Verification items for the finished model (mm, model axes). A direction names the side the tool comes from. Give positions to 0.01 mm unless a question says otherwise; leave off trailing zeros. Write each loop counter-clockwise with the first axis right and the second up, starting at its lowest first coordinate (ties: lowest second). Pieces come first, ordered by that corner, then holes. Notation, with made-up numbers: (33, 84.5) -> (42, 84.5) arc R8 ccw to (42, 93.5) -> close; hole circle Ø7 at (-20, 58). An arc over 180 degrees is marked (long way). Use one line per item in the form item = value. Start each with the question number.
(1) Scan lines: L1, parallel to Y at x = -99.5, z = 10; L2, parallel to X at y = 42.5, z = -20; L3, parallel to Y at x = -99.5, z = 5. Record each from-to range of solid material in increasing order.
(2) Section check B-B, the plane z = -13. State how many separate pieces and enclosed holes the cut face has, plus the area to 3 significant figures.
(3) Depth check by flat-ended pin: pin 1 Ø6 at (y, z) = (33, 0.5) entering from +X; pin 2 Ø2.5 at (x, y) = (-83, 42) entering from -Z; pin 3 Ø5 at (x, z) = (-104.5, 2) entering from +Y; pin 4 Ø2.5 at (y, z) = (43.5, -14) entering from +X. Enter the tip coordinate at first touch or a pass-through.
(4) Set-up check for faces 4 (the face through (-76.171, 42, -17)), 5 (the face through (-88.35, 42.46, 9.86)), 6 (the face through (-64.993, 4.014, -11.003)), 7 (the face through (-104, 2, 8.376)), 8 (the face through (-83, 43, -23.267)): record each of +Z, -Z, +X, -X, +Y, -Y from which the full face is reachable in a straight line by a thin tool's end or side.
(5) Section check D-D, the plane y = 42. Record the cut outline in (x, z).
(6) Release check for a two-part mould opening along Y. For faces 1 (the face through (-66, 3, -14)), 2 (the face through (-103, 2, 13.376)), 3 (the face through (-82, 0, -3)) record: pulls with the +Y half, pulls with the -Y half, needs draft (parallel to the pull), parting line crosses it, or undercut.
from build123d import *

# Parameters (mm, degrees)
AUFSATZ_LINEAR_AUSTRAGEN1_DEPTH  = 5
VERRUNDUNG1_RADIUS               = 2.5
VERRUNDUNG1_LENGTH               = 5
SKIZZE6_W                        = 37
SKIZZE6_H                        = 5
AUFSATZ_LINEAR_AUSTRAGEN3_DEPTH  = 5
SCHNITT_LINEAR_AUSTRAGEN3_DEPTH  = 5
AUFSATZ_LINEAR_AUSTRAGEN6_DEPTH  = 5
SCHNITT_LINEAR_AUSTRAGEN2_DEPTH  = 2
VERRUNDUNG8_RADIUS               = 2.5
VERRUNDUNG8_LENGTH               = 5
VERRUNDUNG9_RADIUS               = 5
VERRUNDUNG9_LENGTH               = 5
SKIZZE37_R                       = 2.5
AUFSATZ_LINEAR_AUSTRAGEN11_DEPTH = 35
SPIEGELN19_START                 = 40
SPIEGELN19_DEPTH                 = 5
SCHNITT_LINEAR_AUSTRAGEN4_DEPTH  = 5
SKIZZE39_W                       = 20
SKIZZE39_H                       = 5
AUFSATZ_LINEAR_AUSTRAGEN12_DEPTH = 5
SKIZZE40_W                       = 17.5
SKIZZE40_H                       = 5
AUFSATZ_LINEAR_AUSTRAGEN14_DEPTH = 5
SKIZZE41_W                       = 17.5
SKIZZE41_H                       = 5
AUFSATZ_LINEAR_AUSTRAGEN15_DEPTH = 5
FASE10_SIZE                      = 5
SKIZZE42_R                       = 1.5
SCHNITT_LINEAR_AUSTRAGEN6_DEPTH  = 127.435665063
SCHNITT_LINEAR_AUSTRAGEN7_DEPTH  = 5


# Read off the part's stored shape, not the designer's step: Spiegeln19
with BuildPart() as part:
    # Skizze2 → Aufsatz-Linear austragen1 (new body)
    with BuildSketch(Plane(origin=(0, 0, 0), x_dir=(1, 0, 0), z_dir=(0, 1, 0))):
        Polygon((-81.170751107, 25.766558824), (-76.170751107, 25.766558824), (-76.170751107, 3.695491012), (-93.241818919, -13.3755768), (-115.312886731, -13.3755768), (-115.312886731, -8.3755768), (-95.312886731, -8.3755768), (-81.170751107, 5.766558824), align=None)
    extrude(amount=AUFSATZ_LINEAR_AUSTRAGEN1_DEPTH)

    # Verrundung1: full round fillet: the end face becomes a half cylinder, R = half its width
    verrundung1_face = Plane((-115.312886731, 2.5, 10.8755768), x_dir=(0, 1, 0), z_dir=(-1, 0, 0))  # on the end face: x along it, z out of the body
    verrundung1_slab = verrundung1_face.offset(-VERRUNDUNG1_RADIUS / 2) * Box(VERRUNDUNG1_LENGTH, 2 * VERRUNDUNG1_RADIUS, VERRUNDUNG1_RADIUS, mode=Mode.PRIVATE)  # the body's end, R deep
    verrundung1_round = Plane((-112.812886731, 2.5, 10.8755768), x_dir=(-1, 0, 0), z_dir=(0, 1, 0)) * Cylinder(VERRUNDUNG1_RADIUS, VERRUNDUNG1_LENGTH, mode=Mode.PRIVATE)  # its axis R under the face
    add(verrundung1_slab - verrundung1_round, mode=Mode.SUBTRACT)

    # Skizze6 → Aufsatz-Linear austragen3 (add, symmetric)
    with BuildSketch(Plane(origin=(-39.933121059, 0, -39.933121059), x_dir=(0.7071067811865485, 0, -0.7071067811865467), z_dir=(0.7071067811865467, 0, 0.7071067811865485))):
        with Locations((-44.818815693, 2.5)):
            Rectangle(SKIZZE6_W, SKIZZE6_H)
    extrude(amount=AUFSATZ_LINEAR_AUSTRAGEN3_DEPTH, both=True)

    # Skizze10 → Schnitt-Linear austragen3 (cut)
    with BuildSketch(Plane.XZ):
        Polygon((-84.706285013, 4.840042894), (-68.089275655, -4.705898652), (-81.170751107, 8.3755768), align=None)
    extrude(amount=-SCHNITT_LINEAR_AUSTRAGEN3_DEPTH, mode=Mode.SUBTRACT)

    # Skizze15 → Aufsatz-Linear austragen6 (add)
    with BuildSketch(Plane.XZ):
        Polygon((-93.241818919, 13.3755768), (-68.089275655, -4.705898652), (-84.706285013, 4.840042894), align=None)
    extrude(amount=-AUFSATZ_LINEAR_AUSTRAGEN6_DEPTH)

    # Skizze9 → Schnitt-Linear austragen2 (cut)
    with BuildSketch(Plane(origin=(0, 5, 0), x_dir=(1, 0, 0), z_dir=(0, 1, 0))):
        with BuildLine():
            Line((-64.90729514, 19.908694448), (-72.710166677, 9.977325168))
            ThreePointArc((-72.710166677, 9.977325168), (-72.613070241, 7.253171877), (-69.888916951, 7.156075442))
            Line((-69.888916951, 7.156075442), (-59.957547671, 14.958946979))
            ThreePointArc((-59.957547671, 14.958946979), (-59.957547671, 19.908694448), (-64.90729514, 19.908694448))
        make_face()
    extrude(amount=-SCHNITT_LINEAR_AUSTRAGEN2_DEPTH, mode=Mode.SUBTRACT)

    # Verrundung8: full round fillet: the end face becomes a half cylinder, R = half its width
    verrundung8_face = Plane((-78.670751107, 2.5, -25.766558824), x_dir=(0, 1, 0), z_dir=(0, 0, -1))  # on the end face: x along it, z out of the body
    verrundung8_slab = verrundung8_face.offset(-VERRUNDUNG8_RADIUS / 2) * Box(VERRUNDUNG8_LENGTH, 2 * VERRUNDUNG8_RADIUS, VERRUNDUNG8_RADIUS, mode=Mode.PRIVATE)  # the body's end, R deep
    verrundung8_round = Plane((-78.670751107, 2.5, -23.266558824), x_dir=(0, 0, -1), z_dir=(0, 1, 0)) * Cylinder(VERRUNDUNG8_RADIUS, VERRUNDUNG8_LENGTH, mode=Mode.PRIVATE)  # its axis R under the face
    add(verrundung8_slab - verrundung8_round, mode=Mode.SUBTRACT)

    # Verrundung9: full round fillet: the end face becomes a half cylinder, R = half its width
    verrundung9_face = Plane((-58.543334109, 2.5, -21.32290801), x_dir=(0, 1, 0), z_dir=(0.707106781187, 0, -0.707106781187))  # on the end face: x along it, z out of the body
    verrundung9_slab = verrundung9_face.offset(-VERRUNDUNG9_RADIUS / 2) * Box(VERRUNDUNG9_LENGTH, 2 * VERRUNDUNG9_RADIUS, VERRUNDUNG9_RADIUS, mode=Mode.PRIVATE)  # the body's end, R deep
    verrundung9_round = Plane((-62.078868015, 2.5, -17.787374104), x_dir=(0.707106781187, 0, -0.707106781187), z_dir=(0, 1, 0)) * Cylinder(VERRUNDUNG9_RADIUS, VERRUNDUNG9_LENGTH, mode=Mode.PRIVATE)  # its axis R under the face
    add(verrundung9_slab - verrundung9_round, mode=Mode.SUBTRACT)

    # Skizze37 → Aufsatz-Linear austragen11 (add)
    with BuildSketch(Plane(origin=(0, 5, 0), x_dir=(1, 0, 0), z_dir=(0, 1, 0))):
        with Locations(Location((-75.486500657, 2.467174327, 0), (0, 0, 305.711324765))):
            Circle(SKIZZE37_R)
    extrude(amount=AUFSATZ_LINEAR_AUSTRAGEN11_DEPTH)

    # Spiegeln19 outline → Spiegeln19 (add)
    with BuildSketch(Plane(origin=(0, 0, 0), x_dir=(1, 0, 0), z_dir=(0, 1, 0)).offset(SPIEGELN19_START)):
        with BuildLine():
            ThreePointArc((-58.543334109, 14.251840198), (-58.543334109, 21.32290801), (-65.614401921, 21.32290801))
            Line((-65.614401921, 21.32290801), (-76.170751107, 10.766558824))
            Line((-76.170751107, 10.766558824), (-76.170751107, 23.266558824))
            ThreePointArc((-76.170751107, 23.266558824), (-78.670751107, 25.766558824), (-81.170751107, 23.266558824))
            Line((-81.170751107, 23.266558824), (-81.170751107, 5.766558824))
            Line((-81.170751107, 5.766558824), (-95.312886731, -8.3755768))
            Line((-95.312886731, -8.3755768), (-112.812886731, -8.3755768))
            ThreePointArc((-112.812886731, -8.3755768), (-115.312886731, -10.8755768), (-112.812886731, -13.3755768))
            Line((-112.812886731, -13.3755768), (-93.241818919, -13.3755768))
            Line((-93.241818919, -13.3755768), (-83.310270003, -6.236057904))
            Line((-83.310270003, -6.236057904), (-81.170751107, -8.3755768))
            Line((-81.170751107, -8.3755768), (-58.543334109, 14.251840198))
        make_face()
    extrude(amount=SPIEGELN19_DEPTH)

    # Skizze38 → Schnitt-Linear austragen4 (cut)
    with BuildSketch(Plane(origin=(0, 45, 0), x_dir=(1, 0, 0), z_dir=(0, 1, 0))):
        Polygon((-83.310270003, -6.236057904), (-69.857042608, 2.938131699), (-81.170751107, -8.3755768), align=None)
    extrude(amount=-SCHNITT_LINEAR_AUSTRAGEN4_DEPTH, mode=Mode.SUBTRACT)

    # Skizze39 → Aufsatz-Linear austragen12 (add)
    with BuildSketch(Plane(origin=(-43.468654965, 0, -43.468654965), x_dir=(-0.7071067811865486, 0, 0.7071067811865465), z_dir=(-0.7071067811865465, 0, -0.7071067811865486))):
        with Locations((63.318815693, 42.5)):
            Rectangle(SKIZZE39_W, SKIZZE39_H)
    extrude(amount=AUFSATZ_LINEAR_AUSTRAGEN12_DEPTH)

    # Skizze40 → Aufsatz-Linear austragen14 (add)
    with BuildSketch(Plane.ZY.offset(81.170751107)):
        with Locations((-14.516558824, 42.5)):
            Rectangle(SKIZZE40_W, SKIZZE40_H)
    extrude(amount=AUFSATZ_LINEAR_AUSTRAGEN14_DEPTH)

    # Skizze41 → Aufsatz-Linear austragen15 (add)
    with BuildSketch(Plane(origin=(0, 0, 8.3755768), x_dir=(-1, 0, 0), z_dir=(0, 0, -1))):
        with Locations((104.062886731, 42.5)):
            Rectangle(SKIZZE41_W, SKIZZE41_H)
    extrude(amount=AUFSATZ_LINEAR_AUSTRAGEN15_DEPTH)

    # Fase10
    fase10_edges = [part.edges().sort_by_distance(p)[0] for p in [
        (-86.170751107, 40, -15.55209273),
        (-91.777352825, 40, -2.231024918),
        (-105.098420637, 40, 3.3755768),
    ]]
    chamfer(fase10_edges, length=FASE10_SIZE - 0.0001)  # a hair under: the kernel refuses the full size

    # Skizze42 → Schnitt-Linear austragen6 (cut, through all)
    with BuildSketch(Plane.XZ):
        with Locations(Location((-62.432421405, -17.433820713, 0), (0, 0, 270))):
            Circle(SKIZZE42_R)
    extrude(amount=-SCHNITT_LINEAR_AUSTRAGEN6_DEPTH, mode=Mode.SUBTRACT)

    # Skizze43 → Schnitt-Linear austragen7 (cut)
    with BuildSketch(Plane(origin=(0, 0, 0), x_dir=(-1, 0, 0), z_dir=(0, -1, 0))):
        Polygon((81.170751107, 5.766558824), (76.170751107, 10.766558824), (76.170751107, 25.766558824), (81.170751107, 25.766558824), align=None)
    extrude(amount=-SCHNITT_LINEAR_AUSTRAGEN7_DEPTH, mode=Mode.SUBTRACT)


solid = part.part
Completed:
q1.L1 = 0 to 5, 40 to 45
q1.L2 = -83.67 to -76.17, -66.94 to -57.6
q1.L3 = 43.38 to 45
q2.separate_pieces = 3
q2.enclosed_holes = 0
q2.area = 163 mm²
q3.pin_1 = -72.99
q3.pin_2 = -23.27
q3.pin_3 = 45
q3.pin_4 = -57.77
q4.face_4 = -Z, +Y, -Y
q4.face_5 = +Z, +X, +Y, -Y
q4.face_6 = none
q4.face_7 = -Z, -X, -Y
q4.face_8 = -Z, -X, +Y, -Y
q5.outline = (-112.81, 6.38) -> (-96.14, 6.38) -> (-83.17, -6.6) -> (-83.17, -23.27) -> (-81.17, -23.27) arc R2.5 ccw to (-76.17, -23.27) -> (-76.17, -10.77) -> (-65.61, -21.32) arc R5 ccw to (-58.54, -14.25) -> (-69.86, -2.94) -> (-83.31, 6.24) -> (-93.24, 13.38) -> (-112.81, 13.38) arc R2.5 ccw to (-112.81, 8.38) -> close; hole circle Ø3 at (-62.43, -17.43)
q6.face_1 = undercut
q6.face_2 = needs draft
q6.face_3 = pulls with the -Y half
